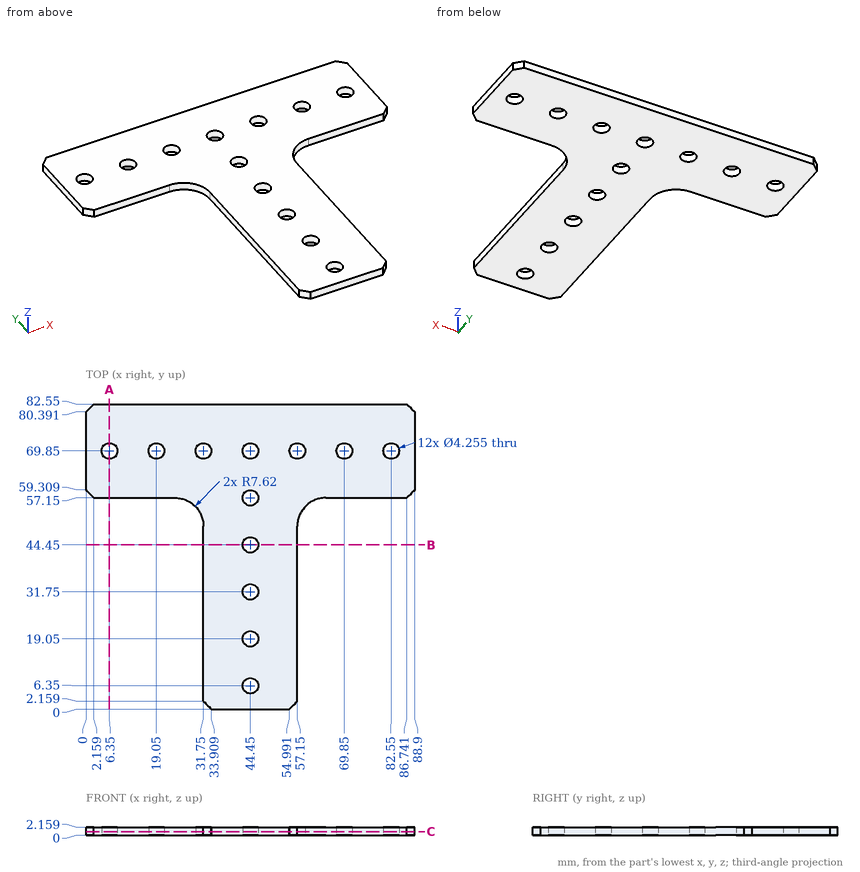
Study the drawing (mm; zero at the part's minimum x, y, z) and answer. Round coordinates to 2 decimals unless told otherwise and drop trailing zeros. Loops run counter-clockwise (first coordinate to the right, second up) from the corner with the lowest first, then second, coordinate; pieces in that order, holes last. Notation, with made-up numbers: (3, 19.5) -> (26, 19.5) arc R18 cw to (26, 34.5) -> close; hole circle Ø5 at (66.5, -12.75). An arc over 180 degrees is marked (long way). Use one line per item in the form item = value.
1. The part is cut by section B-B on y = 44.45. Determine the outline of the cut face in (x, z).
Answer key:
outline = (31.75, 0) -> (42.32, 0) -> (42.32, 2.16) -> (31.75, 2.16) -> close; (46.58, 0) -> (57.15, 0) -> (57.15, 2.16) -> (46.58, 2.16) -> close
2. Find the intervals of material crossed by probe 1 along Y at (x, z) = (82.55, 0.9); probe 2 along X at (y, z) = (36, 1.45); probe 3 along X at (y, z) = (7.5, 0.9), in increasing order. Write a range as [from, to].
Answer key:
probe_1 = [57.15, 67.72], [71.98, 82.55]
probe_2 = [31.75, 57.15]
probe_3 = [31.75, 42.66], [46.24, 57.15]
3. The part is cut by section C-C on z = 0.95. Give the number of separate pieces and of enclosed holes in the cut face, and give its area (3 significant figures).
Answer key:
separate_pieces = 1
enclosed_holes = 12
area = 3,550 mm²
4. A flat-ended cylindrical pin translates along its axis: pin 1 Ø0.6 at (x, z) = (77, 0.5) entering from -Y. Find the tip coordinate at first contact, or state that the pin passes through.
Answer key:
pin_1 = 57.15
5. The part is cut by section A-A on x = 6.35. Determine the outline of the cut face in (y, z).
Answer key:
outline = (57.15, 0) -> (67.72, 0) -> (67.72, 2.16) -> (57.15, 2.16) -> close; (71.98, 0) -> (82.55, 0) -> (82.55, 2.16) -> (71.98, 2.16) -> close
